Verification items for the finished model (mm, model axes). A direction names the side the tool comes from. Round coordinates to 2 decimals unless told otherwise and drop trailing zeros. Order: outer loops, then holes, each group sorted by start corner. A loop starts at its lowest first (then second) coordinate and runs counter-clockwise, first axis right, second up. Notation, with made-up numbers: (87, -1) -> (119, -1) arc R21 ccw to (119, 12) -> close; hole circle Ø7 at (88.5, -6.75). An arc over 180 degrees is marked (long way). Return JSON: item names as keys, results as strings. Group by question number.
Item 1: Scan lines: probe 1 along X at (y, z) = (5.25, -0.5); probe 2 along Y at (x, z) = (3, 5); probe 3 along X at (y, z) = (5.25, 57). Record each from-to range of solid material in increasing order. Write a range as from..to.
Item 2: Sectioned sample at B-B on z = 17. Record the cut outline in (x, y), plus the area to 3 significant figures.
Item 3: Access from +Z, -Z, +X, -X, +Y, -Y to the whole of each face (thin tool, end or side, straight path). Record for faces 4 (the flat face through (7.5, -5, 0)), 5 (the flat face through (-5, -5, -10)), 6 (the flat face through (-1, 5.6, -1)).
Item 4: Sectioned sample at A-A on x = -17. Record the cut outline in (y, z), plus the area to 3 significant figures.
Item 5: Draft check along Z on faces 1 (the flat face through (5, -5, 10)), 2 (the cylindrical face through (48.25, 6.44, -47.69)), 3 (the flat face through (-45.932, 5.194, -45.403)). Enter one of: pulls with the +Z half, pulls with the -Z half, needs draft (parallel to the pull), parting line crosses it, or undercut.
Item 6: Depth check by flat-ended pin: pin 1 Ø4 at (x, y) = (-6, -4.5) entering from -Z; pin 2 Ø3 at (y, z) = (-7, 3.5) entering from +X; pin 3 Ø10 at (x, z) = (18, 7) entering from +Y. Enter the tip coordinate at first touch or a pass-through.
Autodesk Inventor part; units mm, degrees
ref_plane "YZ Plane" through (0, 0, 0) normal (1, 0, 0) x (0, 1, 0)
ref_plane "XZ Plane" through (0, 0, 0) normal (0, 1, 0) x (-1, 0, 0)
ref_plane "XY Plane" through (0, 0, 0) normal (0, 0, 1) x (1, 0, 0)
sketch "스케치3" plane through (0, 0, 0) normal (0, 1, 0) x (-1, 0, 0)
  line L0 (68.1838, -28.2426) -> (28.2426, -68.1838)
  line L1 (28.2426, -68.1838) -> (-28.2426, -68.1838)
  line L2 (-28.2426, -68.1838) -> (-68.1838, -28.2426)
  line L3 (-68.1838, -28.2426) -> (-68.1838, 28.2426)
  line L4 (-68.1838, 28.2426) -> (-28.2426, 68.1838)
  line L5 (-28.2426, 68.1838) -> (28.2426, 68.1838)
  line L6 (28.2426, 68.1838) -> (68.1838, 28.2426)
  line L7 (68.1838, 28.2426) -> (68.1838, -28.2426)
  line L8 (27, -65.1838) -> (-27, -65.1838)
  line L9 (-27, -65.1838) -> (-65.1838, -27)
  line L10 (-65.1838, -27) -> (-65.1838, 27)
  line L11 (-65.1838, 27) -> (-27, 65.1838)
  line L12 (-27, 65.1838) -> (27, 65.1838)
  line L13 (27, 65.1838) -> (65.1838, 27)
  line L14 (65.1838, 27) -> (65.1838, -27)
  line L15 (65.1838, -27) -> (27, -65.1838)
  point P0 (0, 0)
  point P1 (0, 0)
  point P2 (0, 0)
  point P3 (0, 0)
  dimension "d66" = 54
  dimension "d67" = 3
extrude "돌출2" add sketch "스케치3" along normal blind 6.8 contours L0 L1 L2 L3 L4 L5 L6 L7 | L8 L9 L10 L11 L12 L13 L14 L15
sketch "스케치4" plane through (0, 6.8, 0) normal (0, 1, 0) x (1, 0, 0)
  line L0 (26.8343, -64.7838) -> (-26.8343, -64.7838)
  line L1 (-26.8343, -64.7838) -> (-64.7838, -26.8343)
  line L2 (-64.7838, -26.8343) -> (-64.7838, 26.8343)
  line L3 (-64.7838, 26.8343) -> (-26.8343, 64.7838)
  line L4 (-26.8343, 64.7838) -> (26.8343, 64.7838)
  line L5 (26.8343, 64.7838) -> (64.7838, 26.8343)
  line L6 (64.7838, 26.8343) -> (64.7838, -26.8343)
  line L7 (64.7838, -26.8343) -> (26.8343, -64.7838)
  line L8 (-27.5799, 66.5838) -> (27.5799, 66.5838)
  line L9 (27.5799, 66.5838) -> (66.5838, 27.5799)
  line L10 (66.5838, 27.5799) -> (66.5838, -27.5799)
  line L11 (66.5838, -27.5799) -> (27.5799, -66.5838)
  line L12 (27.5799, -66.5838) -> (-27.5799, -66.5838)
  line L13 (-27.5799, -66.5838) -> (-66.5838, -27.5799)
  line L14 (-66.5838, -27.5799) -> (-66.5838, 27.5799)
  line L15 (-66.5838, 27.5799) -> (-27.5799, 66.5838)
  line L16 (-26.7515, 64.5838) -> (26.7515, 64.5838)
  line L17 (26.7515, 64.5838) -> (64.5838, 26.7515)
  line L18 (64.5838, 26.7515) -> (64.5838, -26.7515)
  line L19 (64.5838, -26.7515) -> (26.7515, -64.5838)
  line L20 (26.7515, -64.5838) -> (-26.7515, -64.5838)
  line L21 (-26.7515, -64.5838) -> (-64.5838, -26.7515)
  line L22 (-64.5838, -26.7515) -> (-64.5838, 26.7515)
  line L23 (-64.5838, 26.7515) -> (-26.7515, 64.5838)
  line L24 (-68.1838, 28.2426) -> (-68.1838, -28.2426)
  point P0 (0, 0)
  point P1 (0, 0)
  point P2 (0, 0)
  point P3 (0, 0)
  dimension "d68" = 1.8
  dimension "d69" = 0.2
  dimension "d99" = 1.6
extrude "돌출3" cut sketch "스케치4" against normal blind 2 contours L0 L1 L2 L3 L4 L5 L6 L7 | L8 L9 L10 L11 L12 L13 L14 L15 | L16 L17 L18 L19 L20 L21 L22 L23
sketch "스케치9" plane through (0, 0, 0) normal (0, -1, 0) x (1, 0, 0)
  line L0 (7.5, 10) -> (2.5, 10)
  line L1 (2.5, 10) -> (2.5, -10)
  line L2 (2.5, -10) -> (7.5, -10)
  line L3 (7.5, -10) -> (7.5, 10)
  line L4 (7.5, 10) -> (2.5, -10) construction
  line L5 (2.5, 10) -> (7.5, -10) construction
  line L6 (-2.5, 10) -> (-7.5, 10)
  line L7 (-7.5, 10) -> (-7.5, -10)
  line L8 (-7.5, -10) -> (-2.5, -10)
  line L9 (-2.5, 10) -> (-7.5, -10) construction
  line L10 (-7.5, 10) -> (-2.5, -10) construction
  line L11 (-2.5, -10) -> (-2.5, 10)
  point P0 (0, 0)
  point P1 (5, 0)
  point P2 (-5, 0)
  dimension "d42" = 20
  dimension "d43" = 5
  dimension "d44" = 2.5
  dimension "d47" = 10
extrude "돌출8" add sketch "스케치9" along normal blind 10
sketch "스케치10" plane through (-7.5, 0, -10) normal (-1, 0, 0) x (0, 0, 1)
  circle A0 centre (15, -5) radius 1.25
  line L0 (19.9591, 0) -> (0.0886, 0)
  line L1 (38.2426, 0) -> (-18.2426, 0)
  circle A1 centre (5, -5) radius 1.25
  line L2 (20, 0) -> (20, -10)
  point P0 (10, 0)
  dimension "d54" = 2.5
  dimension "d57" = 10
  dimension "d62" = 5
  dimension "d63" = 5
extrude "돌출9" cut sketch "스케치10" against normal blind 20
sketch "스케치11" plane through (0, 4.8, 0) normal (0, 1, 0) x (1, 0, 0)
  line L0 (-26.7515, 64.5838) -> (26.7515, 64.5838)
  line L1 (26.7515, 64.5838) -> (64.5838, 26.7515)
  line L2 (64.5838, 26.7515) -> (64.5838, -26.7515)
  line L3 (64.5838, -26.7515) -> (26.7515, -64.5838)
  line L4 (26.7515, -64.5838) -> (-26.7515, -64.5838)
  line L5 (-26.7515, -64.5838) -> (-64.5838, -26.7515)
  line L6 (-64.5838, -26.7515) -> (-64.5838, 26.7515)
  line L7 (-64.5838, 26.7515) -> (-26.7515, 64.5838)
  line L8 (-27.5799, 66.5838) -> (27.5799, 66.5838)
  line L9 (-25.5088, 61.5838) -> (25.5088, 61.5838)
  line L10 (25.5088, 61.5838) -> (61.5838, 25.5088)
  line L11 (61.5838, 25.5088) -> (61.5838, -25.5088)
  line L12 (61.5838, -25.5088) -> (25.5088, -61.5838)
  line L13 (25.5088, -61.5838) -> (-25.5088, -61.5838)
  line L14 (-25.5088, -61.5838) -> (-61.5838, -25.5088)
  line L15 (-61.5838, -25.5088) -> (-61.5838, 25.5088)
  line L16 (-61.5838, 25.5088) -> (-25.5088, 61.5838)
  point P0 (0, 0)
  point P1 (0, 0)
  point P2 (0, 0)
  dimension "d70" = 2
  dimension "d71" = 3
extrude "돌출10" add sketch "스케치11" along normal blind 0.8 contours L0 L1 L2 L3 L4 L5 L6 L7 | L9 L10 L11 L12 L13 L14 L15 L16
fillet "모깎기1" radius 1.2 16 edges at (-48.2132, 6.8, 48.2132) (0, 6.8, 68.1838) (48.2132, 6.8, 48.2132) (68.1838, 6.8, 0) (48.2132, 6.8, -48.2132) (0, 6.8, -68.1838) (-48.2132, 6.8, -48.2132) (-68.1838, 6.8, 0) (-48.2132, 0, 48.2132) (0, 0, 68.1838) (48.2132, 0, 48.2132) (68.1838, 0, 0) (48.2132, 0, -48.2132) (0, 0, -68.1838) (-48.2132, 0, -48.2132) (-68.1838, 0, 0)
properties part number "OV-PAM_bottom_2"
Recorded:
{
 "1": {"probe 1": "-68.18..-66.58, -64.58..64.58, 66.58..68.18", "probe 2": "-10..-6.25, -3.75..5.6", "probe 3": "-39.43..-37.16, -34.34..34.34, 37.16..39.43"},
 "2": {"outline": "(-68.18, 1.2) arc R1.2 ccw to (-66.98, 0) -> (66.98, 0) arc R1.2 ccw to (68.18, 1.2) -> (68.18, 5.6) arc R1.2 ccw to (66.98, 6.8) -> (66.58, 6.8) -> (66.58, 4.8) -> (64.58, 4.8) -> (64.58, 5.6) -> (-64.58, 5.6) -> (-64.58, 4.8) -> (-66.58, 4.8) -> (-66.58, 6.8) -> (-66.98, 6.8) arc R1.2 ccw to (-68.18, 5.6) -> close", "area": "763 mm²"},
 "3": {"face 4": "+Z, -Z, +X, -Y", "face 5": "-Z, +X, -X, -Y", "face 6": "+Y"},
 "4": {"outline": "(0, -66.98) arc R1.2 ccw to (1.2, -68.18) -> (5.6, -68.18) arc R1.2 ccw to (6.8, -66.98) -> (6.8, -66.58) -> (4.8, -66.58) -> (4.8, -64.58) -> (5.6, -64.58) -> (5.6, 64.58) -> (4.8, 64.58) -> (4.8, 66.58) -> (6.8, 66.58) -> (6.8, 66.98) arc R1.2 ccw to (5.6, 68.18) -> (1.2, 68.18) arc R1.2 ccw to (0, 66.98) -> close", "area": "763 mm²"},
 "5": {"face 1": "pulls with the +Z half", "face 2": "pulls with the -Z half", "face 3": "undercut"},
 "6": {"pin 1": "z = -10", "pin 2": "x = 7.5", "pin 3": "y = 5.6"}
}
